Verification items for the finished model (mm, model axes). Coordinates: 2 decimals unless noted, no trailing zeros. Order: outer loops, then holes, each group sorted by start corner. A loop starts at its lowest first (then second) coordinate and runs counter-clockwise, first axis right, second up. Notation, with made-up numbers: M -25.75,25 L -17.75,25 A34 ccw -17.75,57 Z; hole C 69.5,2.25 d6. An arc over 180 degrees is marked long. Return JSON: item names as keys, results as strings.
```python
from build123d import *

# Parameters (mm, degrees)
SKETCH_W         = 105
SKETCH_H         = 28.7
PAD_DEPTH        = 2
FILLET_R         = 2.5
HOLE_D           = 3.2
HOLE_DEPTH       = 25
HOLE_CSINK_D     = 6.8
HOLE_CSINK_ANGLE = 90
SKETCH002_W      = 8.8
SKETCH002_H      = 3
SKETCH002_W_2    = 14
SKETCH002_H_2    = 6
SKETCH002_W_3    = 23.5
SKETCH002_H_3    = 6.5
POCKET_DEPTH     = 2.001
FILLET001_R      = 0.75
CHAMFER_SIZE     = 0.5
SKETCH003_R      = 0.975
HOLE001_DEPTH    = 25
SKETCH004_R      = 3
HOLE002_DEPTH    = 25


with BuildPart() as part:
    # Sketch → Pad (new body)
    with BuildSketch(Plane.XZ):
        Rectangle(SKETCH_W, SKETCH_H)
    extrude(amount=-PAD_DEPTH)

    # Fillet
    fillet_edges = [part.edges().sort_by_distance(p)[0] for p in [
        (52.5, 1, 14.35),
        (52.5, 1, -14.35),
        (-52.5, 1, 14.35),
        (-52.5, 1, -14.35),
    ]]
    fillet(fillet_edges, radius=FILLET_R)

    # Hole
    with Locations(Plane.XZ):
        with Locations((46.5, 10.85), (46.5, -10.85), (-46.5, -10.85), (-46.5, 10.85)):
            CounterSinkHole(HOLE_D / 2, HOLE_CSINK_D / 2, depth=HOLE_DEPTH, counter_sink_angle=HOLE_CSINK_ANGLE)

    # Sketch002 → Pocket (cut, through all)
    with BuildSketch(Plane.XZ):
        with Locations((-43, -0.06)):
            Rectangle(SKETCH002_W, SKETCH002_H)
        with Locations((-26, 2.45)):
            Rectangle(SKETCH002_W_2, SKETCH002_H_2)
        with Locations((-8, 2.45)):
            Rectangle(SKETCH002_W_2, SKETCH002_H_2)
        with Locations((19.2, 2.45)):
            Rectangle(SKETCH002_W_3, SKETCH002_H_3)
    extrude(amount=-POCKET_DEPTH, mode=Mode.SUBTRACT)

    # Fillet001
    fillet001_edges = [part.edges().sort_by_distance(p)[0] for p in [
        (-19, 1, -0.55),
        (-1, 1, -0.55),
        (30.95, 1, -0.8),
        (-33, 1, -0.55),
        (-47.4, 1, -1.56),
        (-15, 1, -0.55),
        (7.45, 1, -0.8),
        (-38.6, 1, -1.56),
        (-47.4, 1, 1.44),
        (-33, 1, 5.45),
        (-15, 1, 5.45),
        (7.45, 1, 5.7),
        (30.95, 1, 5.7),
        (-1, 1, 5.45),
        (-19, 1, 5.45),
        (-38.6, 1, 1.44),
    ]]
    fillet(fillet001_edges, radius=FILLET001_R)

    # Chamfer
    chamfer_edges = [part.edges().sort_by_distance(p)[0] for p in [
        (19.2, 0, -0.8),
        (-8, 0, -0.55),
        (-26, 0, -0.55),
        (-43, 0, -1.56),
    ]]
    chamfer(chamfer_edges, length=CHAMFER_SIZE)

    # Sketch003 → Hole001 (cut)
    with BuildSketch(Plane.XZ):
        with Locations((38, 0.94)):
            Circle(SKETCH003_R)
        with Locations((38, 3.48)):
            Circle(SKETCH003_R)
    extrude(amount=-HOLE001_DEPTH, mode=Mode.SUBTRACT)

    # Sketch004 → Hole002 (cut)
    with BuildSketch(Plane.XZ):
        with Locations((46.5, 0)):
            Circle(SKETCH004_R)
    extrude(amount=-HOLE002_DEPTH, mode=Mode.SUBTRACT)


solid = part.part
```
Q1. Cross-section at D-D, the plane y = 1.35. State how many separate pieces and enclosed holes the cut face has, and give its area (3 significant figures).
Values:
{"separate pieces": "1", "enclosed holes": "11", "area": "2,580 mm^2"}
Q2. Cross-section at A-A, the plane x = 38. Record the boundary of the cut face in (y, z) (3 decimals).
Values:
{"outline": "M 0,-14.35 L 2,-14.35 L 2,-0.035 L 0,-0.035 Z; M 0,1.915 L 2,1.915 L 2,2.505 L 0,2.505 Z; M 0,4.455 L 2,4.455 L 2,14.35 L 0,14.35 Z"}
Q3. Material ranges on line 1 along Z through (x, y) = (46.5, 1.9); line 2 along Z through (x, y) = (-46.5, 1.95); line 3 along Z through (x, y) = (38, 1.55) (3 decimals), recorded low to high.
Values:
{"line 1": "-14.35 to -12.45, -9.25 to -3, 3 to 9.25, 12.45 to 14.35", "line 2": "-14.35 to -12.45, -9.25 to -1.56, 1.44 to 9.25, 12.45 to 14.35", "line 3": "-14.35 to -0.035, 1.915 to 2.505, 4.455 to 14.35"}
Q4. Go/stop test with flat-tipped pins: pin 1 (5 mm diameter, centred on x = -46.5, z = 10.85, fed in from -Y); pin 2 (5.5 mm diameter, centred on x = 46.5, z = 0, fed in from +Y). Record where each tip stops, or that it passes through.
Values:
{"pin 1": "y = 0.9", "pin 2": "through"}
Q5. Cross-section at B-B, the plane x = -3. Record the boundary of the cut face in (y, z).
Values:
{"outline": "M 0,-14.35 L 2,-14.35 L 2,-0.55 L 0.5,-0.55 L 0,-1.05 Z; M 0,5.95 L 0.5,5.45 L 2,5.45 L 2,14.35 L 0,14.35 Z"}
Q6. Cross-section at C-C, the plane z = 10.85. Record the boundary of the cut face in (x, y), and give its area (3 significant figures).
Values:
{"outline": "M -52.5,0 L -49.9,0 L -48.1,1.8 L -48.1,2 L -52.5,2 Z; M -44.9,1.8 L -43.1,0 L 43.1,0 L 44.9,1.8 L 44.9,2 L -44.9,2 Z; M 48.1,1.8 L 49.9,0 L 52.5,0 L 52.5,2 L 48.1,2 Z", "area": "191 mm^2"}
Q7. Draft check along Z on faces 1 (the face through (37.026, 0.986, 3.523)), 2 (the face through (-0.7, 2, 0.2)), 3 (the face through (51.787, 1.014, 13.598)), 4 (the face through (43.5, 1, 0.1)). Enter one of: pulls with the +Z half, pulls with the -Z half, needs draft (parallel to the pull), parting line crosses it, or undercut.
Values:
{"face 1": "undercut", "face 2": "needs draft", "face 3": "pulls with the +Z half", "face 4": "undercut"}
